```python
from build123d import *

# Parameters (mm, degrees)
BOSS_EXTRUDE1_DEPTH   = 3.175
F_6_CLEARANCE_HOLE1_D = 4.3053
FILLET3_R             = 1.27
CUT_EXTRUDE3_DEPTH    = 1.778
SKETCH9_W             = 6.096
SKETCH9_H             = 11.176
CUT_EXTRUDE4_DEPTH    = 4.175
SKETCH10_W            = 111.2535
SKETCH10_H            = 8
CUT_EXTRUDE5_DEPTH    = 2.397
FILLET5_R             = 0.508


with BuildPart() as part:
    # Sketch1 → Boss-Extrude1 (new body)
    with BuildSketch(Plane.XY):
        with BuildLine():
            Line((58.7375, -67.1354797), (58.7375, -48.0854797))
            Line((58.7375, -48.0854797), (44.939976119, -39.26086832))
            ThreePointArc((44.939976119, -39.26086832), (40.410479427, -39.106525106), (38.1, -43.0054797))
            Line((38.1, -43.0054797), (38.1, -45.5454797))
            ThreePointArc((38.1, -45.5454797), (37.356051224, -47.341530924), (35.56, -48.0854797))
            Line((35.56, -48.0854797), (-35.56, -48.0854797))
            ThreePointArc((-35.56, -48.0854797), (-37.356051224, -47.341530924), (-38.1, -45.5454797))
            Line((-38.1, -45.5454797), (-38.1, -43.0054797))
            ThreePointArc((-38.1, -43.0054797), (-40.410479427, -39.106525106), (-44.939976119, -39.26086832))
            Line((-44.939976119, -39.26086832), (-58.7375, -48.0854797))
            Line((-58.7375, -48.0854797), (-58.7375, -67.1354797))
            Line((-58.7375, -67.1354797), (58.7375, -67.1354797))
        make_face()
    extrude(amount=BOSS_EXTRUDE1_DEPTH)

    # #6 Clearance Hole1 (through all)
    with Locations(Plane(origin=(0, 0, 0), x_dir=(-1, 0, 0), z_dir=(0, 0, -1))):
        with Locations((42.545, -43.0054797), (-42.545, -43.0054797)):
            Hole(F_6_CLEARANCE_HOLE1_D / 2)

    # Fillet3
    fillet3_edges = [part.edges().sort_by_distance(p)[0] for p in [
        (-58.7375, -67.1354797, 1.5875),
        (-58.7375, -48.0854797, 1.5875),
        (58.7375, -48.0854797, 1.5875),
        (58.7375, -67.1354797, 1.5875),
    ]]
    fillet(fillet3_edges, radius=FILLET3_R)

    # Sketch8 → Cut-Extrude3 (cut)
    with BuildSketch(Plane(origin=(0, 0, 0), x_dir=(-1, 0, 0), z_dir=(0, 0, -1))):
        with BuildLine():
            Line((58.028, -61.8742797), (58.028, -51.3742797))
            ThreePointArc((58.028, -51.3742797), (57.293423807, -49.600855893), (55.52, -48.8662797))
            Line((55.52, -48.8662797), (-55.48, -48.8662797))
            ThreePointArc((-55.48, -48.8662797), (-57.253423807, -49.600855893), (-57.988, -51.3742797))
            Line((-57.988, -51.3742797), (-57.988, -61.8742797))
            ThreePointArc((-57.988, -61.8742797), (-57.253423807, -63.647703507), (-55.48, -64.3822797))
            Line((-55.48, -64.3822797), (55.52, -64.3822797))
            ThreePointArc((55.52, -64.3822797), (57.293423807, -63.647703507), (58.028, -61.8742797))
        make_face()
    extrude(amount=-CUT_EXTRUDE3_DEPTH, mode=Mode.SUBTRACT)

    # Sketch9 → Cut-Extrude4 (cut, through all)
    with BuildSketch(Plane.XY.offset(3.175)):
        with Locations((-25.29, -56.7473797)):
            Rectangle(SKETCH9_W, SKETCH9_H)
        with Locations((25.355, -56.9192547)):
            Rectangle(SKETCH9_W, SKETCH9_H)
    extrude(amount=-CUT_EXTRUDE4_DEPTH, mode=Mode.SUBTRACT)

    # Sketch10 → Cut-Extrude5 (cut, through all)
    with BuildSketch(Plane(origin=(0, 0, 1.778), x_dir=(-1, 0, 0), z_dir=(0, 0, -1))):
        with Locations((0.02, -56.6242797)):
            Rectangle(SKETCH10_W, SKETCH10_H)
    extrude(amount=-CUT_EXTRUDE5_DEPTH, mode=Mode.SUBTRACT)

    # Fillet5
    fillet5_edges = [part.edges().sort_by_distance(p)[0] for p in [
        (-22.242, -51.1593797, 2.4765),
        (-22.242, -62.3353797, 2.4765),
        (-28.338, -62.3353797, 2.4765),
        (-28.338, -51.1593797, 2.4765),
        (28.403, -51.3312547, 2.4765),
        (28.403, -62.5072547, 2.4765),
        (22.307, -62.5072547, 2.4765),
        (22.307, -51.3312547, 2.4765),
        (-28.338, -60.6242797, 2.4765),
        (-28.338, -52.6242797, 2.4765),
        (28.403, -52.6242797, 2.4765),
        (55.60675, -52.6242797, 2.4765),
        (22.307, -52.6242797, 2.4765),
        (-22.242, -52.6242797, 2.4765),
        (28.403, -60.6242797, 2.4765),
        (22.307, -60.6242797, 2.4765),
        (-22.242, -60.6242797, 2.4765),
        (-55.64675, -60.6242797, 2.4765),
        (55.60675, -60.6242797, 2.4765),
        (-55.64675, -52.6242797, 2.4765),
    ]]
    fillet(fillet5_edges, radius=FILLET5_R)


solid = part.part
```
Model file for the job. Use its own axes, mm. A direction names the side the tool comes from. Round coordinates to 2 decimals unless told otherwise and drop trailing zeros. Write each loop counter-clockwise with the first axis right and the second up, starting at its lowest first coordinate (ties: lowest second). Pieces come first, ordered by that corner, then holes. Notation, with made-up numbers: (53, 45.25) - (82, 45.25) arc R14 cw to (82, 63.25) - close; hole circle Ø8 at (64.25, -16). An arc over 180 degrees is marked (long way). Use CSV: the item, a comma, the result in double quotes. Start each with the question number.
Item 1: Two-plate mould, pull along X, no slides. Class faces 4 (the face through (-0.3, -48.5, 0)), 5 (the face through (1, -62, 1.778)), 6 (the face through (58.738, -57, 2)): released by +X, released by -X, zero draft, split by the parting line, or undercut.
Item 2: Drill centre lines: L1, parallel to X at y = -52, z = 2.15; L2, parallel to Y at x = 10, z = 2.6; L3, parallel to X at y = -61, z = 2.2. Where is each one in solid material? Low to high. Write a range as [from, to].
Item 3: Tool access for faces 1 (the face through (-57.31, -49.62, 0.88)), 2 (the face through (51.638, -43.545, 1.565)), 3 (the face through (-38.1, -44, 2)): list every direction of +Z, -Z, +X, -X, +Y, -Y with a clear straight run to the whole face (end or side of a thin tool).
Item 4: Band-saw the part on C-C (z = 1.05). Write the cut outline in (x, y) (1 decimal).
Item 5: Pin check, flat tips, straight feed: P1, Ø5, axis at x = 36, y = -53, coming from the +Z side (3 decimals); P2, Ø0.7, axis at x = 24, z = 2.5, coming from the +Y side. Stop position of each tip, or through.
Item 6: Band-saw the part on A-A (x = -26). Write the cut outline in (y, z) (3 decimals).
Item 7: Band-saw the part on B-B (y = -57.75). Write the cut outline in (x, z) (1 decimal).
Item 8: Band-saw the part on D-D (x = 42.5). Write the cut outline in (y, z) (3 decimals), and give its area (3 significant figures).
Checked values:
1,face 4,"zero draft"
1,face 5,"undercut"
1,face 6,"released by +X"
2,L1,"x = [-58.74, -28.34], [-22.24, 22.31], [28.4, 58.74]"
2,L2,"y = [-67.14, -60.62], [-52.62, -48.09]"
2,L3,"x = [-58.74, -28.36], [-22.22, 22.29], [28.42, 58.74]"
3,face 1,"-Z"
3,face 2,"+Z, -Z, +X, +Y"
3,face 3,"+Z, -Z, +Y"
4,outline,"(-58.7, -65.9) arc R1.3 ccw to (-57.5, -67.1) - (57.5, -67.1) arc R1.3 ccw to (58.7, -65.9) - (58.7, -48.8) arc R1.3 ccw to (58.2, -47.7) - (44.9, -39.3) arc R4.4 ccw to (38.1, -43) - (38.1, -45.5) arc R2.5 cw to (35.6, -48.1) - (-35.6, -48.1) arc R2.5 cw to (-38.1, -45.5) - (-38.1, -43) arc R4.4 ccw to (-44.9, -39.3) - (-58.2, -47.7) arc R1.3 ccw to (-58.7, -48.8) - close; hole (-58, -61.9) arc R2.5 ccw to (-55.5, -64.4) - (55.5, -64.4) arc R2.5 ccw to (58, -61.9) - (58, -51.4) arc R2.5 ccw to (55.5, -48.9) - (-55.5, -48.9) arc R2.5 ccw to (-58, -51.4) - close; hole circle Ø4.3 at (-42.5, -43); hole circle Ø4.3 at (42.5, -43)"
5,P1,"stops at z = 3.175"
5,P2,"stops at y = -48.09"
6,outline,"(-67.135, 0) - (-64.382, 0) - (-64.382, 1.778) - (-62.335, 1.778) - (-62.335, 3.175) - (-67.135, 3.175) - close; (-51.159, 1.778) - (-48.866, 1.778) - (-48.866, 0) - (-48.085, 0) - (-48.085, 3.175) - (-51.159, 3.175) - close"
7,outline,"(-58.7, 0) - (-58, 0) - (-58, 1.8) - (-55.6, 1.8) - (-55.6, 3.2) - (-58.7, 3.2) - close; (55.6, 1.8) - (58, 1.8) - (58, 0) - (58.7, 0) - (58.7, 3.2) - (55.6, 3.2) - close"
8,outline,"(-67.135, 0) - (-64.382, 0) - (-64.382, 1.778) - (-60.624, 1.778) - (-60.624, 3.175) - (-67.135, 3.175) - close; (-52.624, 1.778) - (-48.866, 1.778) - (-48.866, 0) - (-45.158, 0) - (-45.158, 3.175) - (-52.624, 3.175) - close; (-40.853, 0) - (-38.561, 0) - (-38.561, 3.175) - (-40.853, 3.175) - close"
8,area,"38.3 mm²"
